```python
from build123d import *

# Parameters (mm, degrees)
SKETCH1_W           = 200
SKETCH1_H           = 20
SKETCH1_W_2         = 4.6
SKETCH1_H_2         = 10.2
SKETCH1_W_3         = 4.55
SKETCH1_H_3         = 10.1
SKETCH1_W_4         = 4.5
SKETCH1_H_4         = 10
SKETCH1_W_5         = 4.45
SKETCH1_H_5         = 9.9
SKETCH1_W_6         = 4.4
SKETCH1_H_6         = 9.8
SKETCH1_W_7         = 4.35
SKETCH1_H_7         = 9.7
SKETCH1_W_8         = 4.3
SKETCH1_H_8         = 9.6
SKETCH1_W_9         = 4.25
SKETCH1_H_9         = 9.5
SKETCH1_W_10        = 4.2
SKETCH1_H_10        = 9.4
SKETCH1_W_11        = 4.15
SKETCH1_H_11        = 9.3
BOSS_EXTRUDE1_DEPTH = 4.5


with BuildPart() as part:
    # Sketch1 → Boss-Extrude1 (new body)
    with BuildSketch(Plane(origin=(0, 0, 0), x_dir=(1, 0, 0), z_dir=(0, 1, 0))):
        Rectangle(SKETCH1_W, SKETCH1_H)
        with Locations((-80, 0)):
            Rectangle(SKETCH1_W_2, SKETCH1_H_2, mode=Mode.SUBTRACT)
        with Locations((-62, 0)):
            Rectangle(SKETCH1_W_3, SKETCH1_H_3, mode=Mode.SUBTRACT)
        with Locations((-44, 0)):
            Rectangle(SKETCH1_W_4, SKETCH1_H_4, mode=Mode.SUBTRACT)
        with Locations((-26, 0)):
            Rectangle(SKETCH1_W_5, SKETCH1_H_5, mode=Mode.SUBTRACT)
        with Locations((-8, 0)):
            Rectangle(SKETCH1_W_6, SKETCH1_H_6, mode=Mode.SUBTRACT)
        with Locations((10, 0)):
            Rectangle(SKETCH1_W_7, SKETCH1_H_7, mode=Mode.SUBTRACT)
        with Locations((28, 0)):
            Rectangle(SKETCH1_W_8, SKETCH1_H_8, mode=Mode.SUBTRACT)
        with Locations((46, 0)):
            Rectangle(SKETCH1_W_9, SKETCH1_H_9, mode=Mode.SUBTRACT)
        with Locations((64, 0)):
            Rectangle(SKETCH1_W_10, SKETCH1_H_10, mode=Mode.SUBTRACT)
        with Locations((82, 0)):
            Rectangle(SKETCH1_W_11, SKETCH1_H_11, mode=Mode.SUBTRACT)
    extrude(amount=BOSS_EXTRUDE1_DEPTH)


solid = part.part
```
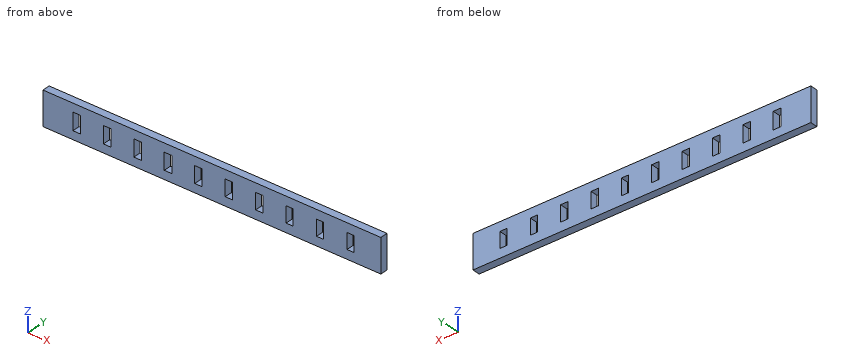
Read the model definition and answer for the solid it produces. Units are mm, in the model's axes. Round coordinates to 2 decimals unless told otherwise and drop trailing zeros. Use CSV: the item, a comma, the result in double quotes.
Q1. This flat-tipped pin is pushed along its axis until it touches: pin 1 Ø2 at (x, z) = (-23.5, 3) entering from -Y. Where does it stop, or does it pass through?
Values:
pin 1,"stops at y = 0"
Q2. Straight lines are drawn through the part: line 1 along Z through (x, y) = (-45.5, 0.7); line 2 along Z through (x, y) = (45, 2.35). For each, find the intervals that lie inside material, in ascending order.
Values:
line 1,"z = -10 to -5, 5 to 10"
line 2,"z = -10 to -4.75, 4.75 to 10"
Q3. Find section A-A, the plane z = 2. Count the separate pieces of the cut face and the enclosed holes in it, then the cut area to 3 significant figures.
Values:
separate pieces,"11"
enclosed holes,"0"
area,"703 mm²"
